Geometry check sheet. Reference: drawing and pictorial views, mm from the part's lowest x, y, z. Give positions to 0.01 mm unless a question says otherwise; leave off trailing zeros. Write each loop counter-clockwise with the first axis right and the second up, starting at its lowest first coordinate (ties: lowest second). Pieces come first, ordered by that corner, then holes. Notation, with made-up numbers: (89, 12) - (104, 12) arc R29 ccw to (104, 39) - close; hole circle Ø8 at (-1, -7.75). An arc over 180 degrees is marked (long way). Write item = value, one per line. Start each with the question number.
(1) Section check D-D, the plane x = 18. Enter the section's corners in (y, z), plus the area to 3 significant figures.
(2) Thickness scan on L1, parallel to Z at x = 80.5, y = 2.95; L2, parallel to X at y = 4.3, z = 28; L3, parallel to Z at x = 194, y = 2.05. Record the ranges inside material, lowest first.
(3) Section check A-A, the plane z = 6. Enter the section's corners in (x, y).
(4) Section check C-C, the plane z = 68.5. Enter the section's corners in (x, y), plus the area to 3 significant figures.
(5) Section check B-B, the plane x = 150. Enter the section's corners in (y, z), plus the area to 3 significant figures.
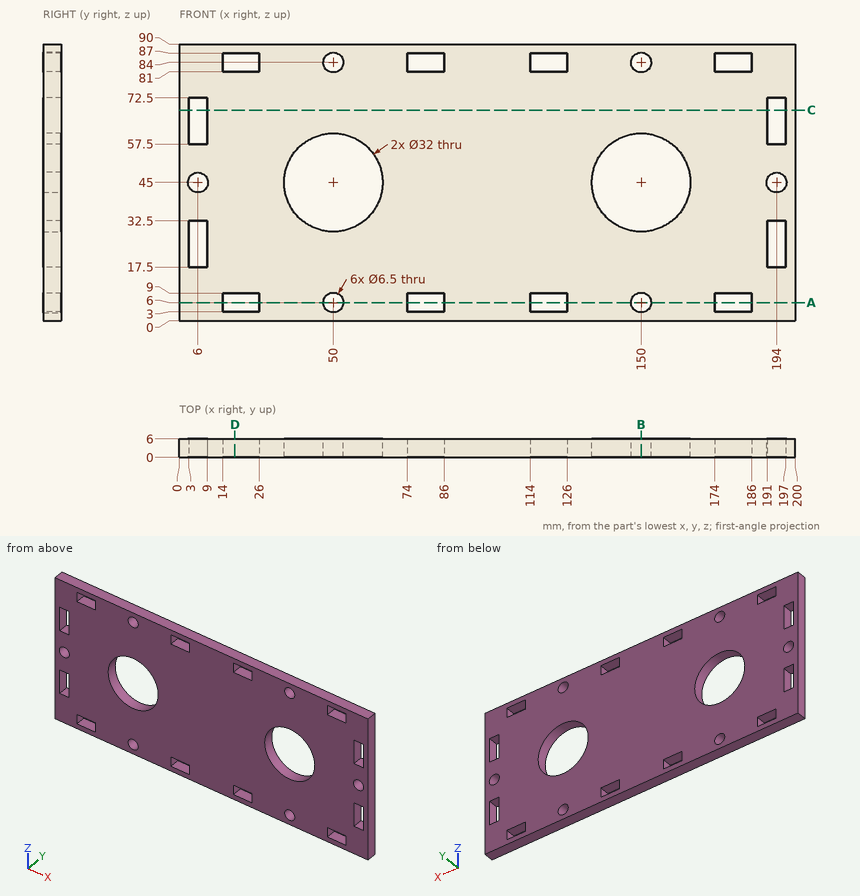
Model answer:
q1.outline = (0, 0) - (6, 0) - (6, 3) - (0, 3) - close; (0, 9) - (6, 9) - (6, 81) - (0, 81) - close; (0, 87) - (6, 87) - (6, 90) - (0, 90) - close
q1.area = 468 mm²
q2.L1 = 0 to 3, 9 to 81, 87 to 90
q2.L2 = 0 to 3, 9 to 191, 197 to 200
q2.L3 = 0 to 17.5, 32.5 to 41.75, 48.25 to 57.5, 72.5 to 90
q3.outline = (0, 0) - (14, 0) - (14, 6) - (0, 6) - close; (26, 0) - (46.75, 0) - (46.75, 6) - (26, 6) - close; (53.25, 0) - (74, 0) - (74, 6) - (53.25, 6) - close; (86, 0) - (114, 0) - (114, 6) - (86, 6) - close; (126, 0) - (146.75, 0) - (146.75, 6) - (126, 6) - close; (153.25, 0) - (174, 0) - (174, 6) - (153.25, 6) - close; (186, 0) - (200, 0) - (200, 6) - (186, 6) - close
q4.outline = (0, 0) - (3, 0) - (3, 6) - (0, 6) - close; (9, 0) - (191, 0) - (191, 6) - (9, 6) - close; (197, 0) - (200, 0) - (200, 6) - (197, 6) - close
q4.area = 1,130 mm²
q5.outline = (0, 0) - (6, 0) - (6, 2.75) - (0, 2.75) - close; (0, 9.25) - (6, 9.25) - (6, 29) - (0, 29) - close; (0, 61) - (6, 61) - (6, 80.75) - (0, 80.75) - close; (0, 87.25) - (6, 87.25) - (6, 90) - (0, 90) - close
q5.area = 270 mm²
